Geometry check sheet. Reference: the model listing, model coordinates, mm. Face numbers are marked on the shaded views. A direction names the side the tool comes from. Round coordinates to 2 decimals unless told otherwise and drop trailing zeros. Write each loop counter-clockwise with the first axis right and the second up, starting at its lowest first coordinate (ties: lowest second). Pieces come first, ordered by that corner, then holes. Notation, with made-up numbers: M 75.25,36.5 L 101.25,36.5 A18 cw 101.25,55.5 Z; hole C 27,23 d6. An arc over 180 degrees is marked long. Use a Markdown table: item, result.
```python
from build123d import *

# Parameters (mm, degrees)
SKETCH1_R           = 18.415
BOSS_EXTRUDE1_DEPTH = 23.876
SKETCH2_R           = 5.9055
BOSS_EXTRUDE2_DEPTH = 5.588
SKETCH3_R           = 2.921
BOSS_EXTRUDE3_DEPTH = 14.859
SKETCH4_R           = 17.0815
BOSS_EXTRUDE4_DEPTH = 30.48
SKETCH5_R           = 16.891
BOSS_EXTRUDE5_DEPTH = 15.24
SKETCH6_R           = 1.143
CUT_EXTRUDE1_DEPTH  = 15.24
CIRPATTERN1_COUNT   = 2
SKETCH8_W           = 14.224
SKETCH8_H           = 3.683
CUT_EXTRUDE2_DEPTH  = 2.54


with BuildPart() as part:
    # Sketch1 → Boss-Extrude1 (new body)
    with BuildSketch(Plane.XY):
        Circle(SKETCH1_R)
    extrude(amount=-BOSS_EXTRUDE1_DEPTH)

    # Sketch2 → Boss-Extrude2 (add)
    with BuildSketch(Plane.XY):
        with Locations((0, -8.636)):
            Circle(SKETCH2_R)
    extrude(amount=BOSS_EXTRUDE2_DEPTH)

    # Sketch3 → Boss-Extrude3 (add)
    with BuildSketch(Plane.XY.offset(5.588)):
        with Locations((0, -8.636)):
            Circle(SKETCH3_R)
    extrude(amount=BOSS_EXTRUDE3_DEPTH)

    # Sketch4 → Boss-Extrude4 (add)
    with BuildSketch(Plane(origin=(0, 0, -23.876), x_dir=(-1, 0, 0), z_dir=(0, 0, -1))):
        Circle(SKETCH4_R)
    extrude(amount=BOSS_EXTRUDE4_DEPTH)

    # Sketch5 → Boss-Extrude5 (add)
    with BuildSketch(Plane(origin=(0, 0, -54.356), x_dir=(-1, 0, 0), z_dir=(0, 0, -1))):
        Circle(SKETCH5_R)
    extrude(amount=BOSS_EXTRUDE5_DEPTH)

    # Sketch6 → Cut-Extrude1 (cut)
    with BuildSketch(Plane.XY):
        with Locations((7.871883333, -13.049561402)):
            Circle(SKETCH6_R)
        with Locations((15.24, 0)):
            Circle(SKETCH6_R)
        with Locations((7.871883333, 13.049561402)):
            Circle(SKETCH6_R)
    cut_extrude1 = extrude(amount=-CUT_EXTRUDE1_DEPTH, mode=Mode.SUBTRACT)

    # CirPattern1: Cut-Extrude1 ×2 about axis
    cirpattern1_axis = Axis((0, 0, 0), (0, 0, 1))
    for i in range(1, CIRPATTERN1_COUNT):
        add(cut_extrude1.rotate(cirpattern1_axis, i * 360 / CIRPATTERN1_COUNT), mode=Mode.SUBTRACT)

    # Sketch8 → Cut-Extrude2 (cut)
    with BuildSketch(Plane(origin=(0, -16.891, 0), x_dir=(-1, 0, 0), z_dir=(0, -1, 0))):
        with Locations((0, 58.7375)):
            Rectangle(SKETCH8_W, SKETCH8_H)
    extrude(amount=-CUT_EXTRUDE2_DEPTH, mode=Mode.SUBTRACT)


solid = part.part
```
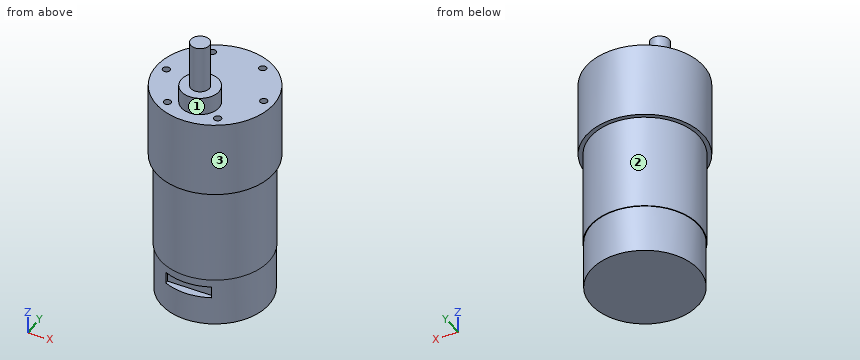
Item 1: Cross-section at C-C, the plane z = -14. Record the cut outline in (x, y) (3 decimals).
Outcome:
| item | result |
|---|---|
| outline | C 0,0 d36.83; hole C -15.24,0 d2.286; hole C -7.872,-13.05 d2.286; hole C -7.872,13.05 d2.286; hole C 7.872,-13.05 d2.286; hole C 7.872,13.05 d2.286; hole C 15.24,0 d2.286 |
Item 2: Access from +Z, -Z, +X, -X, +Y, -Y to the whole of each face (thin tool, end or side, straight path). Record for the marked faces 1, 2 and 3.
Outcome:
| item | result |
|---|---|
| face 1 | +Z |
| face 2 | -Z |
| face 3 | +Z, -Z |
Item 3: Go/stop test with flat-tipped pins: pin 1 (1.1 mm diameter, centred on y = -15, z = -58, fed in from +X); pin 2 (1 mm diameter, centred on x = -12.5, z = 0, fed in from -Y); pin 3 (3 mm diameter, centred on x = 2.5, z = -58.5, fed in from -Y). Record where each tip stops, or that it passes through.
Outcome:
| item | result |
|---|---|
| pin 1 | stops at x = 8.75 |
| pin 2 | stops at y = -13.97 |
| pin 3 | stops at y = -14.35 |
Item 4: Material ranges on line 1 along X through (y, z) = (-13, -4); line 2 along Z through (x, y) = (-13.5, -12); line 3 along Z through (x, y) = (15, 1.5), recorded low to high. Write a range as from..to.
Outcome:
| item | result |
|---|---|
| line 1 | x = -13.04..-9.01, -6.73..6.73, 9.01..13.04 |
| line 2 | z = -23.88..0 |
| line 3 | z = -69.6..0 |
Item 5: Cross-section at D-D, the plane z = -59. Record the cut outline in (x, y).
Outcome:
| item | result |
|---|---|
| outline | M -7.11,-15.32 L -7.11,-14.35 L 7.11,-14.35 L 7.11,-15.32 A16.89 ccw long Z |
